```python
from build123d import *

# Parameters (mm, degrees)
F1_DEPTH = 25


with BuildPart() as f1:
    # F0 (on Top) → F1 (new body)
    with BuildSketch(Plane.XY):
        with BuildLine():
            ThreePointArc((0, -23.013084), (-10.622454, -16.666771), (-10.068095, -4.305342))
            ThreePointArc((-10.068095, -4.305342), (-10.163555, 4.074881), (-4.305342, 10.068095))
            ThreePointArc((-4.305342, 10.068095), (-16.666771, 10.622454), (-23.013084, 0))
            ThreePointArc((-23.013084, 0), (-16.272708, -16.272708), (0, -23.013084))
        make_face()
        with BuildLine():
            ThreePointArc((8.884421, 6.400748), (9.533999, 5.385662), (10.068095, 4.305342))
            ThreePointArc((10.068095, 4.305342), (10.622454, 16.666771), (0, 23.013084))
            ThreePointArc((0, 23.013084), (-16.272708, 16.272708), (-23.013084, 0))
            ThreePointArc((-23.013084, 0), (-16.666771, 10.622454), (-4.305342, 10.068095))
            ThreePointArc((-4.305342, 10.068095), (2.933317, 10.549794), (8.884421, 6.400748))
        make_face()
        with BuildLine():
            ThreePointArc((23.013084, 0), (16.666771, -10.622454), (4.305342, -10.068095))
            ThreePointArc((4.305342, -10.068095), (-4.074881, -10.163555), (-10.068095, -4.305342))
            ThreePointArc((-10.068095, -4.305342), (-10.622454, -16.666771), (0, -23.013084))
            ThreePointArc((0, -23.013084), (16.272708, -16.272708), (23.013084, 0))
        make_face()
        with BuildLine():
            ThreePointArc((10.068095, 4.305342), (10.727258, 2.197369), (10.95, 0))
            ThreePointArc((10.95, 0), (9.139092, -6.031542), (4.305342, -10.068095))
            ThreePointArc((4.305342, -10.068095), (16.666771, -10.622454), (23.013084, 0))
            ThreePointArc((23.013084, 0), (16.272708, 16.272708), (0, 23.013084))
            ThreePointArc((0, 23.013084), (10.622454, 16.666771), (10.068095, 4.305342))
        make_face()
    extrude(amount=F1_DEPTH)


solid = f1.part
```
Input: part model. Units: mm. Frame: model coordinates. A direction names the side the tool comes from. Coordinates: 2 decimals unless noted, no trailing zeros. Loops run counter-clockwise (first coordinate to the right, second up) from the corner with the lowest first, then second, coordinate; pieces in that order, holes last. Notation, with made-up numbers: (-31.75, 51) -> (3.25, 51) arc R9 ccw to (3.25, 65) -> close; hole circle Ø11 at (1, -25.5). An arc over 180 degrees is marked (long way). Use a Markdown table: item, result.
1) Material intervals for line 1 along X through (y, z) = (6.5, 14.5); line 2 along X through (y, z) = (5.5, 21); line 3 along Y through (x, z) = (8.5, 9.25), sorted ascending. Write a range as from..to.
Results found:
| item | result |
|---|---|
| line 1 | x = -22.08..-8.81, 8.81..22.08 |
| line 2 | x = -22.35..-9.47, 9.47..22.35 |
| line 3 | y = -21.39..-6.9, 6.9..21.39 |
2) Cut plane A-A (x = -6.5). Return the cut outline in (y, z), then the cut area to 3 significant figures.
Results found:
| item | result |
|---|---|
| outline | (-22.08, 0) -> (-8.81, 0) -> (-8.81, 25) -> (-22.08, 25) -> close; (8.81, 0) -> (22.08, 0) -> (22.08, 25) -> (8.81, 25) -> close |
| area | 663 mm2 |
3) Cut plane C-C (z = 5.25). Return the cut outline in (x, y), then the cut area to 3 significant figures.
Results found:
| item | result |
|---|---|
| outline | (-23.01, 0) arc R23.01 ccw to (0, -23.01) arc R23.01 ccw to (23.01, 0) arc R23.01 ccw to (0, 23.01) arc R23.01 ccw to start; hole (-4.31, 10.07) arc R10.95 ccw (long way) to (10.95, 0) arc R10.95 ccw to (10.07, 4.31) arc R10.95 ccw to (8.88, 6.4) arc R10.95 ccw to start |
| area | 1,290 mm2 |
4) Access query for faces 3 (the flat face through (5, -10, 0)), 4 (the cylindrical face through (9.526, 5.4, 12.325)). Directions: +Z, -Z, +X, -X, +Y, -Y. A direction counts if a zero-diameter tool reaches every point of the face in a straight line with its end or side. Return the directions, or none.
Results found:
| item | result |
|---|---|
| face 3 | -Z, +X, -X, +Y, -Y |
| face 4 | +Z, -Z |
5) Cut plane B-B (y = 5). Return the cut outline in (x, z).
Results found:
| item | result |
|---|---|
| outline | (-22.46, 0) -> (-9.74, 0) -> (-9.74, 25) -> (-22.46, 25) -> close; (9.74, 0) -> (22.46, 0) -> (22.46, 25) -> (9.74, 25) -> close |
6) Pull-direction query (X, two-part tool) for faces 1 (the cylindrical face through (10.72, 2.23, 12.32)), 2 (the flat face through (5, -10, 25)); classes: released by +X, released by -X, zero draft, split by the parting line, or undercut.
Results found:
| item | result |
|---|---|
| face 1 | undercut |
| face 2 | zero draft |
7) Contact query for flat-ended pins moving along their axis: pin 1 (3 mm diameter, centred on y = 8, z = 18.5, fed in from -X); pin 2 (5 mm diameter, centred on x = 6.5, z = 20.5, fed in from +Y). Output: stop coordinate, or through.
Results found:
| item | result |
|---|---|
| pin 1 | stops at x = -22.08 |
| pin 2 | stops at y = 22.66 |
8) Cut plane D-D (x = 20). Return the cut outline in (y, z).
Results found:
| item | result |
|---|---|
| outline | (-11.38, 0) -> (11.38, 0) -> (11.38, 25) -> (-11.38, 25) -> close |
